Check sheet for the modelled part. Datum: model origin and axes. Units: mm. A direction names the side the tool comes from. Round coordinates to 2 decimals unless told otherwise and drop trailing zeros. Write each loop counter-clockwise with the first axis right and the second up, starting at its lowest first coordinate (ties: lowest second). Pieces come first, ordered by that corner, then holes. Notation, with made-up numbers: M 13,-20 L 29,-20 A30 cw 29,4 Z; hole C 83.5,45.25 d6. An arc over 180 degrees is marked long. One line per item, written item: value.
from build123d import *

# Parameters (mm, degrees)
F2_R     = 8.5
F3_DEPTH = 14
F4_R     = 2.4
F5_R     = 5


with BuildPart() as f1:
    # F0 (on Front) → F1 (revolve)
    with BuildSketch(Plane.XZ):
        with BuildLine():
            Line((0, 100), (0, 0))
            Line((0, 0), (25.5, 0))
            Line((25.5, 0), (25.5, 83))
            ThreePointArc((25.5, 83), (20.520815, 95.020815), (8.5, 100))
            Line((8.5, 100), (0, 100))
        make_face()
    revolve(axis=Axis((0, 0, 50), (0, 0, -1)))

    # F2 (on face) → F3 (join)
    with BuildSketch(Plane.XY.offset(100)):
        Circle(F2_R)
    extrude(amount=F3_DEPTH)

    # F4
    f4_edges = [f1.edges().sort_by_distance(p)[0] for p in [
        (-8.5, 0, 114),
    ]]
    fillet(f4_edges, radius=F4_R)

    # F5
    f5_edges = [f1.edges().sort_by_distance(p)[0] for p in [
        (-25.5, 0, 0),
    ]]
    fillet(f5_edges, radius=F5_R)


solid = f1.part
Q1. Scan lines: line 1 (X direction, y = -1, z = 47); line 2 (X direction, y = -3.5, z = 78.5); line 3 (Z direction, x = 3.5, y = 21). Record each from-to range of solid material in increasing order. Write a range as [from, to].
Completed:
line 1: [-25.48, 25.48]
line 2: [-25.26, 25.26]
line 3: [0.06, 94.2]
Q2. Access from +Z, -Z, +X, -X, +Y, -Y to the whole of each face (thin tool, end or side, straight path). Record for faces 1 (the flat face through (0, 0, 0)), 2 (the cylindrical face through (4.57, 7.167, 105.719)).
Completed:
face 1: -Z, +X, -X, +Y, -Y
face 2: +Z
Q3. Sectioned sample at A-A on z = 80. Enter the section's corners in (x, y), and give its area (3 significant figures).
Completed:
outline: C 0,0 d51
area: 2,040 mm^2
Q4. Depth check by flat-ended pin: P1, Ø1.5, axis at x = -6.5, z = 40.5, coming from the +Y side; P2, Ø3, axis at x = -11, z = 86.5, coming from the +Y side; P3, Ø12, axis at x = -19.5, y = 8, coming from the +Z side. Enter the tip coordinate at first touch or a pass-through.
Completed:
P1: y = 24.84
P2: y = 23.34
P3: z = 98.68
